For this review, take the finished solid that the model builds, in its own axes (mm). Give positions to 0.01 mm unless a question says otherwise; leave off trailing zeros. Order: outer loops, then holes, each group sorted by start corner. A loop starts at its lowest first (then second) coordinate and runs counter-clockwise, first axis right, second up. Notation, with made-up numbers: M 33.25,31 L 85.25,31 A19 ccw 85.25,61 Z; hole C -29,70.25 d8. An arc over 180 degrees is marked long. Answer as CSV lines item,"result". Start each with the question number.
1. For line 1 along X through (y, z) = (2, 5); line 2 along X through (y, z) = (-8.5, 4); line 3 along Z through (x, y) = (20, -0.5), list the stretches that pass through material, from the lowest coordinate up.
2. We need section A-A, the plane y = 3. Give the boundary of the cut face in (x, z), and give its area (3 significant figures).
3. Mouldability with a two-part tool opening along X and no side actions: class faces 1 (the cylindrical face through (204.516, -5.285, -1.727)), 2 (the flat face through (113, 7, 24.047)), 3 (the flat face through (230, -5, -1)) as pulls with the +X half, pulls with the -X half, needs draft (parallel to the pull), parting line crosses it, or undercut.
4. We need section C-C, the plane x = 20. Give the boundary of the cut face in (y, z), and give its area (3 significant figures).
5. Clearance check with flat-ended pins moving along their axes: P1, Ø10, axis at x = 82, y = -6, coming from the -Z side; P2, Ø2, axis at x = 195, y = -15, coming from the -Z side; P3, Ø3, axis at x = 53.5, y = -17.5, coming from the +Z side. State where each tip first meets the part, or that it passes through.
6. We need section B-B, the plane z = 0. Give the boundary of the cut face in (x, y).
7. We need section D-D, the plane x = 102. Give the boundary of the cut face in (y, z), and give its area (3 significant figures).
from build123d import *

# Parameters (mm, degrees)
BOSS_EXTRUDE1_DEPTH          = 230
F_11_5_11_5_DIAMETER_HOLE2_D = 11.5


with BuildPart() as part:
    # Sketch1 → Boss-Extrude1 (new body)
    with BuildSketch(Plane(origin=(0, 0, 0), x_dir=(0, 0, -1), z_dir=(1, 0, 0))):
        with BuildLine():
            Line((-24.046920821, 0), (-24.046920821, 15))
            Line((-24.046920821, 15), (25.953079179, 15))
            Line((25.953079179, 15), (25.953079179, 0))
            ThreePointArc((25.953079179, 0), (0.953079179, -25), (-24.046920821, 0))
        make_face()
    extrude(amount=BOSS_EXTRUDE1_DEPTH)

    # Ø11.5 (11.5) Diameter Hole2 (through all)
    with Locations(Plane(origin=(0, 15, 0), x_dir=(1, 0, 0), z_dir=(0, 1, 0))):
        with Locations((20, 0), (210, 0)):
            Hole(F_11_5_11_5_DIAMETER_HOLE2_D / 2)


solid = part.part
Result set:
1,line 1,"0 to 17.16, 22.84 to 207.16, 212.84 to 230"
1,line 2,"0 to 15.87, 24.13 to 205.87, 214.13 to 230"
1,line 3,"-25.95 to -5.75, 5.75 to 24.04"
2,outline,"M 0,-25.95 L 230,-25.95 L 230,24.05 L 0,24.05 Z; hole C 20,0 d11.5; hole C 210,0 d11.5"
2,area,"11,300 mm2"
3,face 1,"undercut"
3,face 2,"needs draft"
3,face 3,"pulls with the +X half"
4,outline,"M -24.54,-5.75 A25 ccw 0,-25.95 L 15,-25.95 L 15,-5.75 Z; M -24.08,5.75 L 15,5.75 L 15,24.05 L 0,24.05 A25 ccw Z"
4,area,"1,270 mm2"
5,P1,"z = -25.93"
5,P2,"z = -21.67"
5,P3,"z = 18.26"
6,outline,"M 0,-24.98 L 14.25,-24.98 L 14.25,15 L 0,15 Z; M 25.75,-24.98 L 204.25,-24.98 L 204.25,15 L 25.75,15 Z; M 215.75,-24.98 L 230,-24.98 L 230,15 L 215.75,15 Z"
7,outline,"M 0,-25.95 L 15,-25.95 L 15,24.05 L 0,24.05 A25 ccw Z"
7,area,"1,730 mm2"
